CAD build for the part. Positions are in the model's coordinates, mm. Face numbers are marked on the shaded views. A direction names the side the tool comes from. Round coordinates to 2 decimals unless told otherwise and drop trailing zeros. Loops run counter-clockwise (first coordinate to the right, second up) from the corner with the lowest first, then second, coordinate; pieces in that order, holes last. Notation, with made-up numbers: (-39, -2) -> (-23, -2) arc R16 cw to (-23, 5) -> close; hole circle Ø6 at (19, 36). An arc over 180 degrees is marked (long way). Answer as CSV lines item,"result".
```python
from build123d import *

# Parameters (mm, degrees)
F0_W     = 200
F0_H     = 18
F0_R     = 2
F1_DEPTH = 2
F2_W     = 200
F2_H     = 2.4
F3_DEPTH = 25
F4_W     = 200
F4_H     = 22.8
F5_DEPTH = 3


with BuildPart() as f1:
    # F0 (on Top) → F1 (new body)
    with BuildSketch(Plane.XY):
        with Locations((100, 9)):
            Rectangle(F0_W, F0_H)
        with Locations((5, 9)):
            Circle(F0_R, mode=Mode.SUBTRACT)
        with BuildLine():
            Line((12, 11), (93, 11))
            ThreePointArc((93, 11), (95, 9), (93, 7))
            Line((93, 7), (12, 7))
            ThreePointArc((12, 7), (10, 9), (12, 11))
        make_face(mode=Mode.SUBTRACT)
        with Locations((100, 9)):
            Circle(F0_R, mode=Mode.SUBTRACT)
        with BuildLine():
            Line((107, 11), (188, 11))
            ThreePointArc((188, 11), (190, 9), (188, 7))
            Line((188, 7), (107, 7))
            ThreePointArc((107, 7), (105, 9), (107, 11))
        make_face(mode=Mode.SUBTRACT)
        with Locations((195, 9)):
            Circle(F0_R, mode=Mode.SUBTRACT)
    extrude(amount=F1_DEPTH)

    # F2 (on face) → F3 (join)
    with BuildSketch(Plane(origin=(0, 0, 0), x_dir=(1, 0, 0), z_dir=(0, 0, -1))):
        with Locations((100, 1.2)):
            Rectangle(F2_W, F2_H)
        with Locations((100, -19.2)):
            Rectangle(F2_W, F2_H)
    extrude(amount=-F3_DEPTH)

    # F4 (on face) → F5 (join)
    with BuildSketch(Plane(origin=(0, 0, 0), x_dir=(1, 0, 0), z_dir=(0, 0, -1))):
        with Locations((100, -9)):
            Rectangle(F4_W, F4_H)
    extrude(amount=F5_DEPTH)


solid = f1.part
```
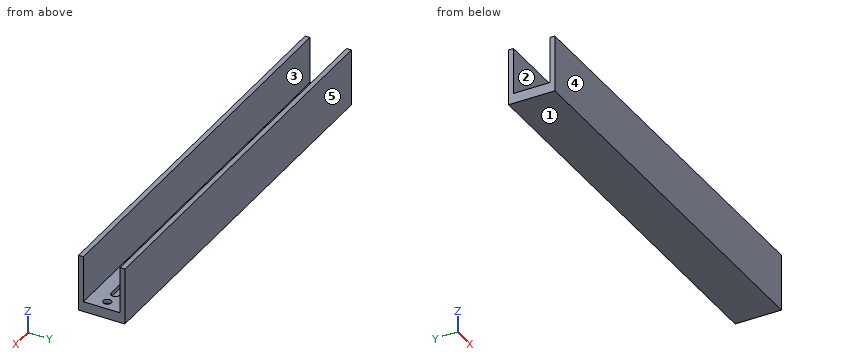
Q1. Slice it at B-B, the plane x = 100. Give the cut face in (y, z).
Results:
outline,"(-2.4, -3) -> (20.4, -3) -> (20.4, 25) -> (18, 25) -> (18, 2) -> (11, 2) -> (11, 0) -> (7, 0) -> (7, 2) -> (0, 2) -> (0, 25) -> (-2.4, 25) -> close"
Q2. Two-plate mould, pull along Y, no slides. Class the marked faces 3, 4 and 5: pulls with the +Y half, pulls with the -Y half, needs draft (parallel to the pull), parting line crosses it, or undercut.
Results:
face 3,"undercut"
face 4,"pulls with the -Y half"
face 5,"pulls with the +Y half"
Q3. Slice it at A-A, the plane z = 7.5. Give the cut face in (x, y), and give its area (3 significant figures).
Results:
outline,"(0, -2.4) -> (200, -2.4) -> (200, 0) -> (0, 0) -> close; (0, 18) -> (200, 18) -> (200, 20.4) -> (0, 20.4) -> close"
area,"960 mm2"
Q4. Drop flat-ended pins along their axis: pin 1 Ø5.5 at (x, y) = (121, 4.5) entering from +Z; pin 2 Ø1.2 at (x, y) = (99, 9.5) entering from +Z. Give the stop position or say it passes through.
Results:
pin 1,"z = 2"
pin 2,"z = 0"
Q5. Tool access for the marked faces 1 and 2: list every direction of +Z, -Z, +X, -X, +Y, -Y with a clear straight run to the whole face (end or side of a thin tool).
Results:
face 1,"-Z, +X, -X, +Y, -Y"
face 2,"+Z, +X, -X"
Q6. Probe L1, parallel to Y at x = 195, z = 0.65; L2, parallel to Y at x = 39, z = 6.75; L3, parallel to Z at x = 31, y = 4. List the from-to ranges inside material, lowest first. Write a range as [from, to].
Results:
L1,"[-2.4, 7], [11, 20.4]"
L2,"[-2.4, 0], [18, 20.4]"
L3,"[-3, 2]"
Q7. Slice it at C-C, the plane y = 13.25. Give the cut face in (x, z).
Results:
outline,"(0, -3) -> (200, -3) -> (200, 2) -> (0, 2) -> close"
